Design review of the part built by this model. Coordinates are the model's own, in mm. A direction names the side the tool comes from. Round coordinates to 2 decimals unless told otherwise and drop trailing zeros. Write each loop counter-clockwise with the first axis right and the second up, starting at its lowest first coordinate (ties: lowest second). Pieces come first, ordered by that corner, then holes. Notation, with made-up numbers: (24, -16.5) -> (58, -16.5) arc R29 ccw to (58, 3.5) -> close; hole circle Ø2 at (67.5, 12). An arc over 180 degrees is marked (long way). One line per question, with ' | ' between items. Start each with the question number.
1) For probe 1 along Y at (x, z) = (0.75, 44); probe 2 along Y at (x, z) = (2.75, 81), list the stretches that pass through material, from the lowest coordinate up.
2) Consider section B-B (y = 0). Give the boundary of the cut face in (x, z), then the cut area to 3 significant figures.
3) Consider section D-D (z = 21.5). Give the boundary of the cut face in (x, y).
4) Mouldability with a two-part tool opening along Y and no side actions: class faces 1 (the flat face through (-8, 3, 78)), 2 (the cylindrical face through (-5, 1.6, 34.5)), 3 (the cylindrical face through (1.37, -10.41, 44.86)) as +Y half, -Y half, draft (parallel to the pull), parting line (faces both ways), or undercut.
5) Consider section A-A (z = 81). Give the boundary of the cut face in (x, y), then the cut area to 3 significant figures.
6) Consider section C-C (x = 0). Give the boundary of the cut face in (y, z), then the cut area to 3 significant figures.
7) For faces 4 (the flat face through (-9, 0, 68)), 5 (the flat face through (0, 0, 93)), 6 (the flat face through (2.5, -4.8, 0)), 7 (the flat face through (9, 0, 68)), 8 (the flat face through (0, 0, 70)), list the 3-axis set-ups (+Z, -Z, +X, -X, +Y, -Y) from which the entire face can be reached by the end or side of a thin tool; tool diameter is ignored.
8) Insertion check: pin 1 Ø7 at (y, z) = (0, 78) entering from +X; pin 2 Ø0.8 at (x, y) = (-8.5, -0.5) entering from +Z; pin 3 Ø6 at (y, z) = (-6, 68.5) entering from -X. Each pin has a flat end and moves straight along its axis. Give the tip position at first contact, or say it passes through.
```python
from build123d import *

# Parameters (mm, degrees)
SKETCH_1_R          = 10.5
EXTRUDE_1_DEPTH     = 93
SKETCH_2_R          = 5.25
CUT_EXTRUDE_2_DEPTH = 70
FILLET_1_R          = 2
SKETCH_3_W          = 11
SKETCH_3_H          = 25
CUT_EXTRUDE_3_DEPTH = 15
SKETCH_4_R          = 4
CUT_EXTRUDE_4_DEPTH = 15


with BuildPart() as part:
    # Эскиз1 → Вытянуть1 (new body)
    with BuildSketch(Plane.XY):
        with Locations(Location((0, 0, 0), (0, 0, 180))):
            Circle(SKETCH_1_R)
    extrude(amount=EXTRUDE_1_DEPTH)

    # Эскиз2 → Вытянуть2 (cut)
    with BuildSketch(Plane(origin=(0, 0, 0), x_dir=(-1, 0, 0), z_dir=(0, 0, -1))):
        Circle(SKETCH_2_R)
    extrude(amount=-CUT_EXTRUDE_2_DEPTH, mode=Mode.SUBTRACT)

    # Скругление1
    fillet_1_edges = [part.edges().sort_by_distance(p)[0] for p in [
        (10.5, 0, 93),
    ]]
    fillet(fillet_1_edges, radius=FILLET_1_R)

    # Эскиз3 → Вытянуть3 (cut, symmetric)
    with BuildSketch(Plane(origin=(0, 0, 0), x_dir=(1, 0, 0), z_dir=(0, 1, 0))):
        with Locations((-13.5, -80.5)):
            Rectangle(SKETCH_3_W, SKETCH_3_H)
        with Locations((13.5, -80.5)):
            Rectangle(SKETCH_3_W, SKETCH_3_H)
    extrude(amount=CUT_EXTRUDE_3_DEPTH, both=True, mode=Mode.SUBTRACT)

    # Эскиз4 → Вытянуть4 (cut, symmetric)
    with BuildSketch(Plane(origin=(0, 0, 0), x_dir=(0, 0, -1), z_dir=(1, 0, 0))):
        with Locations((-81, 0)):
            Circle(SKETCH_4_R)
    extrude(amount=CUT_EXTRUDE_4_DEPTH, both=True, mode=Mode.SUBTRACT)


solid = part.part
```
From the geometry:
1) probe 1: y = -10.47 to -5.2, 5.2 to 10.47 | probe 2: y = -10.13 to -4, 4 to 10.13
2) outline: (-10.5, 0) -> (-5.25, 0) -> (-5.25, 70) -> (5.25, 70) -> (5.25, 0) -> (10.5, 0) -> (10.5, 68) -> (8, 68) -> (8, 77) -> (-8, 77) -> (-8, 68) -> (-10.5, 68) -> close; (-8, 85) -> (8, 85) -> (8, 93) -> (-8, 93) -> close | area: 965 mm2
3) outline: circle Ø21 at (0, 0); hole circle Ø10.5 at (0, 0)
4) face 1: draft | face 2: undercut | face 3: parting line
5) outline: (-8, -6.8) arc R10.5 ccw to (8, -6.8) -> (8, -4) -> (-8, -4) -> close; (-8, 4) -> (8, 4) -> (8, 6.8) arc R10.5 ccw to (-8, 6.8) -> close | area: 172 mm2
6) outline: (-10.5, 0) -> (-5.25, 0) -> (-5.25, 70) -> (5.25, 70) -> (5.25, 0) -> (10.5, 0) -> (10.5, 91) arc R2 ccw to (8.5, 93) -> (-8.5, 93) arc R2 ccw to (-10.5, 91) -> close; hole circle Ø8 at (0, 81) | area: 1,170 mm2
7) face 4: +Z, -X, +Y, -Y | face 5: +Z, +X, -X, +Y, -Y | face 6: -Z, +X, -X, +Y, -Y | face 7: +Z, +X, +Y, -Y | face 8: -Z
8) pin 1: stops at x = 8 | pin 2: stops at z = 68 | pin 3: stops at x = -10.05
